```python
from build123d import *

# Parameters (mm, degrees)
SKETCH2_W           = 80
SKETCH2_H           = 50
BOSS_EXTRUDE1_DEPTH = 40
SKETCH3_W           = 68
SKETCH3_H           = 38
CUT_EXTRUDE1_DEPTH  = 6
DRAFT1_START        = -34
DRAFT1_DEPTH        = 68
DRAFT1_START_2      = -20
DRAFT1_2_DEPTH      = 40


with BuildPart() as part:
    # Sketch2 → Boss-Extrude1 (new body)
    with BuildSketch(Plane(origin=(0, 0, 0), x_dir=(1, 0, 0), z_dir=(0, 1, 0))):
        Rectangle(SKETCH2_W, SKETCH2_H)
    extrude(amount=BOSS_EXTRUDE1_DEPTH)

    # Sketch3 → Cut-Extrude1 (cut)
    with BuildSketch(Plane.XZ):
        Rectangle(SKETCH3_W, SKETCH3_H)
    extrude(amount=-CUT_EXTRUDE1_DEPTH, mode=Mode.SUBTRACT)

    # Draft1: read off the stored shape, not the designer's step
    # Draft1 outline → Draft1 (add)
    with BuildSketch(Plane.YZ.offset(DRAFT1_START)):
        Polygon((6, 19), (0, 19), (6, 15.535898385), align=None)
        Polygon((6, -19), (6, -15.535898385), (0, -19), align=None)
    extrude(amount=DRAFT1_DEPTH)

    # Draft1 2 outline → Draft1 2 (add)
    with BuildSketch(Plane.XY.offset(DRAFT1_START_2)):
        Polygon((34, 6), (30.535898385, 6), (34, 0), align=None)
        Polygon((-34, 0), (-30.535898385, 6), (-34, 6), align=None)
    extrude(amount=DRAFT1_2_DEPTH)


solid = part.part
```
The model under review builds one solid part; all positions refer to its coordinate system, in mm. A direction names the side the tool comes from. Round coordinates to 2 decimals unless told otherwise and drop trailing zeros. Loops run counter-clockwise (first coordinate to the right, second up) from the corner with the lowest first, then second, coordinate; pieces in that order, holes last.
Item 1: Take a section at A-A (x = 26). Write out the cut boundary in (y, z), then the cut area to 3 significant figures.
Determined:
outline: (0, -25) - (40, -25) - (40, 25) - (0, 25) - (0, 19) - (6, 15.54) - (6, -15.54) - (0, -19) - close
area: 1,790 mm2
Item 2: Mouldability with a two-part tool opening along Z and no side actions: class faces 1 (the face through (-1, 20, 25)), 2 (the face through (-0.48, 2.96, 17.29)), 3 (the face through (40, 20, 0)), 4 (the face through (-32.29, 2.96, -0.27)) as released by +Z, released by -Z, zero draft, split by the parting line, or undercut.
Determined:
face 1: released by +Z
face 2: undercut
face 3: zero draft
face 4: undercut
Item 3: For line 1 (Y direction, x = 7, z = 10.5); line 2 (Z direction, x = -31, y = 3); line 3 (Y direction, x = 26.5, z = -18), list the stretches that pass through material, from the lowest coordinate up.
Determined:
line 1: y = 6 to 40
line 2: z = -25 to -17.27, 17.27 to 25
line 3: y = 1.73 to 40
Item 4: Take a section at C-C (z = -13.5). Write out the cut boundary in (x, y), then the cut area to 3 significant figures.
Determined:
outline: (-40, 0) - (-34, 0) - (-30.54, 6) - (30.54, 6) - (34, 0) - (40, 0) - (40, 40) - (-40, 40) - close
area: 2,810 mm2
Item 5: For faces 5 (the face through (-1, 40, 0)), 6 (the face through (32.244, 3.042, -0.266)), list the 3-axis set-ups (+Z, -Z, +X, -X, +Y, -Y) from which the entire face can be reached by the end or side of a thin tool; tool diameter is ignored.
Determined:
face 5: +Z, -Z, +X, -X, +Y
face 6: -Y
Item 6: Take a section at B-B (y = 5). Write out the cut boundary in (x, z), then the cut area to 3 significant figures.
Determined:
outline: (-40, -25) - (40, -25) - (40, 25) - (-40, 25) - close; hole (-31.11, -16.11) - (31.11, -16.11) - (31.11, 16.11) - (-31.11, 16.11) - close
area: 1,990 mm2
Item 7: Clearance check with a flat-ended pin moving along its axis: pin 1 Ø3 at (x, z) = (8.5, 1) entering from -Y. State where the tip first meets the part, or that it passes through.
Determined:
pin 1: stops at y = 6
